For this review, take the finished solid that the model builds, in its own axes (mm). A direction names the side the tool comes from. Round coordinates to 2 decimals unless told otherwise and drop trailing zeros. Write each loop counter-clockwise with the first axis right and the second up, starting at its lowest first coordinate (ties: lowest second). Pieces come first, ordered by that corner, then holes. Notation, with made-up numbers: M 33.25,38.5 L 86.25,38.5 A26 ccw 86.25,67.5 Z; hole C 28.25,84 d4. An arc over 180 degrees is marked long. One line per question, with ' | ' between items.
```python
from build123d import *

# Parameters (mm, degrees)
SKETCH_1_W           = 200
SKETCH_1_H           = 54
SKETCH_1_R           = 2.1
EXTRUDE_1_DEPTH      = 3
SKETCH_3_W           = 200
SKETCH_3_H           = 14
EXTRUDE_2_DEPTH      = 3
SKETCH_2_R           = 1.6
CUT_EXTRUDE_1_DEPTH  = 10
EXTRUDE_3_DEPTH      = 3
SKETCH_5_W           = 26.5
SKETCH_5_H           = 42
CUT_EXTRUDE_2_DEPTH  = 10
FILLET_1_R           = 15
FILLET_2_R           = 2
SKETCH_14_W          = 79
SKETCH_14_H          = 57
CUT_EXTRUDE_7_DEPTH  = 10
CHAMFER_1_SIZE       = 12
FILLET_4_R           = 5
SKETCH_15_W          = 15
SKETCH_15_H          = 57
SKETCH_15_W_2        = 10.75
SKETCH_15_H_2        = 35
CUT_EXTRUDE_10_DEPTH = 10
FILLET_5_R           = 2
SKETCH_16_W          = 52.508149225
SKETCH_16_H          = 7.45
SKETCH_16_W_2        = 5.991850775
CUT_EXTRUDE_11_DEPTH = 10
FILLET_6_R           = 2
SKETCH_17_R          = 1.55
CUT_EXTRUDE_12_DEPTH = 10
SKETCH_18_R          = 1.55
CUT_EXTRUDE_13_DEPTH = 10


with BuildPart() as part:
    # 草图1 → 凸台-拉伸1 (new body)
    with BuildSketch(Plane.XY):
        Rectangle(SKETCH_1_W, SKETCH_1_H)
        with Locations((-47.5, 21)):
            Circle(SKETCH_1_R, mode=Mode.SUBTRACT)
        with Locations((-47.5, 4)):
            Circle(SKETCH_1_R, mode=Mode.SUBTRACT)
        with Locations((-47.5, -21)):
            Circle(SKETCH_1_R, mode=Mode.SUBTRACT)
        with Locations(Location((47.5, -21, 0), (0, 0, 180))):
            Circle(SKETCH_1_R, mode=Mode.SUBTRACT)
        with Locations(Location((47.5, 4, 0), (0, 0, 180))):
            Circle(SKETCH_1_R, mode=Mode.SUBTRACT)
        with Locations(Location((47.5, 21, 0), (0, 0, 180))):
            Circle(SKETCH_1_R, mode=Mode.SUBTRACT)
    extrude(amount=EXTRUDE_1_DEPTH)

    # 草图3 → 凸台-拉伸2 (add)
    with BuildSketch(Plane.XY.offset(3)):
        with Locations((0, -34)):
            Rectangle(SKETCH_3_W, SKETCH_3_H)
    extrude(amount=-EXTRUDE_2_DEPTH)

    # 草图2 → 切除-拉伸1 (cut)
    with BuildSketch(Plane.XY.offset(3)):
        with Locations((59, 9.5)):
            Circle(SKETCH_2_R)
        with Locations((77.5, 9.5)):
            Circle(SKETCH_2_R)
        with Locations((77.5, -35.5)):
            Circle(SKETCH_2_R)
        with Locations((59, -35.5)):
            Circle(SKETCH_2_R)
    extrude(amount=-CUT_EXTRUDE_1_DEPTH, mode=Mode.SUBTRACT)

    # 草图4 → 凸台-拉伸3 (add)
    with BuildSketch(Plane.XY.offset(3)):
        Polygon((-100, 30), (-100, 27), (100, 27), (100, -41), (120, -41), (120, 30), align=None)
    extrude(amount=-EXTRUDE_3_DEPTH)

    # 草图5 → 切除-拉伸2 (cut)
    with BuildSketch(Plane.XY.offset(3)):
        with Locations((106.75, -10.45)):
            Rectangle(SKETCH_5_W, SKETCH_5_H)
    extrude(amount=-CUT_EXTRUDE_2_DEPTH, mode=Mode.SUBTRACT)

    # 圆角1
    fillet_1_edges = [part.edges().sort_by_distance(p)[0] for p in [
        (93.5, -31.45, 1.5),
        (93.5, 10.55, 1.5),
    ]]
    fillet(fillet_1_edges, radius=FILLET_1_R)

    # 圆角2
    fillet_2_edges = [part.edges().sort_by_distance(p)[0] for p in [
        (-100, -41, 1.5),
        (120, -41, 1.5),
        (120, 30, 1.5),
        (-100, 30, 1.5),
        (120, 10.55, 1.5),
        (120, -31.45, 1.5),
    ]]
    fillet(fillet_2_edges, radius=FILLET_2_R)

    # 草图14 → 切除-拉伸7 (cut)
    with BuildSketch(Plane(origin=(0, 0, 0), x_dir=(-1, 0, 0), z_dir=(0, 0, -1))):
        with Locations((0, -6.5)):
            Rectangle(SKETCH_14_W, SKETCH_14_H)
    extrude(amount=-CUT_EXTRUDE_7_DEPTH, mode=Mode.SUBTRACT)

    # 倒角1
    chamfer_1_edges = [part.edges().sort_by_distance(p)[0] for p in [
        (-39.5, 22, 1.5),
        (-39.5, -35, 1.5),
        (39.5, -35, 1.5),
        (39.5, 22, 1.5),
    ]]
    chamfer(chamfer_1_edges, length=CHAMFER_1_SIZE)

    # 圆角4
    fillet_4_edges = [part.edges().sort_by_distance(p)[0] for p in [
        (27.5, 22, 1.5),
        (-27.5, 22, 1.5),
        (-39.5, -23, 1.5),
        (-39.5, 10, 1.5),
        (27.5, -35, 1.5),
        (-27.5, -35, 1.5),
        (39.5, 10, 1.5),
        (39.5, -23, 1.5),
    ]]
    fillet(fillet_4_edges, radius=FILLET_4_R)

    # 草图15 → 切除-拉伸10 (cut)
    with BuildSketch(Plane(origin=(0, 0, 0), x_dir=(-1, 0, 0), z_dir=(0, 0, -1))):
        with Locations((65.5, -6.5)):
            Rectangle(SKETCH_15_W, SKETCH_15_H)
        with Locations((84.5, -6.5)):
            Rectangle(SKETCH_15_W, SKETCH_15_H)
        with Locations((-60.875, -13)):
            Rectangle(SKETCH_15_W_2, SKETCH_15_H_2)
        with Locations((-75.625, -13)):
            Rectangle(SKETCH_15_W_2, SKETCH_15_H_2)
    extrude(amount=-CUT_EXTRUDE_10_DEPTH, mode=Mode.SUBTRACT)

    # 圆角5
    fillet_5_edges = [part.edges().sort_by_distance(p)[0] for p in [
        (70.25, 4.5, 1.5),
        (70.25, -30.5, 1.5),
        (81, -30.5, 1.5),
        (81, 4.5, 1.5),
        (66.25, 4.5, 1.5),
        (55.5, 4.5, 1.5),
        (55.5, -30.5, 1.5),
        (66.25, -30.5, 1.5),
        (-92, -35, 1.5),
        (-77, -35, 1.5),
        (-77, 22, 1.5),
        (-92, 22, 1.5),
        (-58, 22, 1.5),
        (-73, 22, 1.5),
        (-73, -35, 1.5),
        (-58, -35, 1.5),
    ]]
    fillet(fillet_5_edges, radius=FILLET_5_R)

    # 草图16 → 切除-拉伸11 (cut)
    with BuildSketch(Plane(origin=(0, 0, 0), x_dir=(-1, 0, 0), z_dir=(0, 0, -1))):
        with Locations((-87.745925387, 20.275)):
            Rectangle(SKETCH_16_W, SKETCH_16_H)
        with Locations((-58.495925388, 20.275)):
            Rectangle(SKETCH_16_W_2, SKETCH_16_H)
    extrude(amount=-CUT_EXTRUDE_11_DEPTH, mode=Mode.SUBTRACT)

    # 圆角6
    fillet_6_edges = [part.edges().sort_by_distance(p)[0] for p in [
        (55.5, 16.55, 1.5),
        (114, 16.55, 1.5),
        (114, 24, 1.5),
        (55.5, 24, 1.5),
    ]]
    fillet(fillet_6_edges, radius=FILLET_6_R)

    # 草图17 → 切除-拉伸12 (cut)
    with BuildSketch(Plane(origin=(0, 0, 0), x_dir=(-1, 0, 0), z_dir=(0, 0, -1))):
        with Locations((-7.5, 26)):
            Circle(SKETCH_17_R)
        with Locations((12.5, 26)):
            Circle(SKETCH_17_R)
    extrude(amount=-CUT_EXTRUDE_12_DEPTH, mode=Mode.SUBTRACT)

    # 草图18 → 切除-拉伸13 (cut)
    with BuildSketch(Plane(origin=(0, 0, 0), x_dir=(-1, 0, 0), z_dir=(0, 0, -1))):
        with Locations((97, 12.5)):
            Circle(SKETCH_18_R)
        with Locations((97, -7.5)):
            Circle(SKETCH_18_R)
    extrude(amount=-CUT_EXTRUDE_13_DEPTH, mode=Mode.SUBTRACT)


solid = part.part
```
Item 1: Machinability: for faces 1 (the face through (98.01, 6.27, 1.48)), 2 (the face through (33.4, 16.1, 1.5)), 3 (the face through (33, 19, 3)), which of the approach directions +Z, -Z, +X, -X, +Y, -Y give a long, thin tool a straight path to every point of the face, cutting with its end or side? Answer none if there is none.
Results:
face 1: +Z, -Z, +X | face 2: +Z, -Z | face 3: +Z, +X, -X, +Y, -Y
Item 2: Take a section at C-C (x = 47.5). Write out the cut boundary in (y, z), then the cut area to 3 significant figures.
Results:
outline: M -41,0 L -23.1,0 L -23.1,3 L -41,3 Z; M -18.9,0 L 1.9,0 L 1.9,3 L -18.9,3 Z; M 6.1,0 L 18.9,0 L 18.9,3 L 6.1,3 Z; M 23.1,0 L 30,0 L 30,3 L 23.1,3 Z | area: 175 mm2
Item 3: Insertion check: pin 1 Ø1.5 at (y, z) = (-9.5, 1.5) entering from +X; pin 2 Ø10 at (x, y) = (87, -22) entering from -Z; pin 3 Ø0.9 at (y, z) = (-1.5, 2) entering from +X; pin 4 Ø4 at (x, y) = (-47.5, 21) entering from +Z. Each pin has a flat end and moves straight along its axis. Give the tip position at first contact, or say it passes through.
Results:
pin 1: x = 93.5 | pin 2: z = 0 | pin 3: x = 93.89 | pin 4: through
Item 4: Take a section at B-B (x = -36). Write out the cut boundary in (y, z), then the cut area to 3 significant figures.
Results:
outline: M -41,0 L -26.5,0 L -26.5,3 L -41,3 Z; M 13.5,0 L 30,0 L 30,3 L 13.5,3 Z | area: 93.0 mm2
Item 5: To check wall thickness, follow line 1 along Y through (x, z) = (73, 0.25); line 2 along Y through (x, z) = (-12.5, 1.9); line 3 along X through (y, z) = (-4, 0.25). State the ranges of each line that lie inside material, in increasing order. Write a range as from..to.
Results:
line 1: -41..-30.5, 4.5..16.55, 24..30 | line 2: -41..-35, 22..24.45, 27.55..30 | line 3: -100..-92, -77..-73, -58..-39.5, 39.5..55.5, 66.25..70.25, 81..93.51
Item 6: Take a section at A-A (y = -13). Write out the cut boundary in (x, z), then the cut area to 3 significant figures.
Results:
outline: M -100,0 L -92,0 L -92,3 L -100,3 Z; M -77,0 L -73,0 L -73,3 L -77,3 Z; M -58,0 L -39.5,0 L -39.5,3 L -58,3 Z; M 39.5,0 L 55.5,0 L 55.5,3 L 39.5,3 Z; M 66.25,0 L 70.25,0 L 70.25,3 L 66.25,3 Z; M 81,0 L 93.5,0 L 93.5,3 L 81,3 Z | area: 189 mm2
Item 7: Mouldability with a two-part tool opening along X and no side actions: class faces 4 (the face through (97.78, -26.94, 1.48)), 5 (the face through (33, 19, 0)), 6 (the face through (-33.6, 15.9, 1.5)) as +X half, -X half, draft (parallel to the pull), parting line (faces both ways), or undercut.
Results:
face 4: +X half | face 5: draft | face 6: undercut
Item 8: Take a section at D-D (z = 1.9). State how many separate pieces and enclosed holes the cut face has, then the cut area to 3 significant figures.
Results:
separate pieces: 1 | enclosed holes: 20 | area: 7,360 mm2
